Input: part model. Units: mm. Frame: model coordinates. A direction names the side the tool comes from. Round coordinates to 2 decimals unless told otherwise and drop trailing zeros. Order: outer loops, then holes, each group sorted by start corner. A loop starts at its lowest first (then second) coordinate and runs counter-clockwise, first axis right, second up. Notation, with made-up numbers: (-16.75, 58.25) - (-6.75, 58.25) arc R21 ccw to (-6.75, 64.25) - close; hole circle Ø6 at (57.25, -35.5). An arc over 180 degrees is marked (long way). One line per item, written item: value. Start each with the question number.
from build123d import *

# Parameters (mm, degrees)
SKETCH2_R           = 5.55625
BOSS_EXTRUDE1_DEPTH = 15
CHAMFER1_SIZE       = 0.5


with BuildPart() as part:
    # Sketch1 → Revolve1 (revolve)
    with BuildSketch(Plane(origin=(0, 0, 0), x_dir=(1, 0, 0), z_dir=(0, 1, 0))):
        Polygon((1, 25), (2, 25), (2, 15), (7.9375, 15), (7.9375, 0), (5.55625, 0), (5.55625, 12), (1, 12), align=None)
    revolve(axis=Axis((0, 0, 0), (0, 0, -1)))

    # Sketch2 → Boss-Extrude1 (add, through all)
    with BuildSketch(Plane(origin=(0, 0, -15), x_dir=(-1, 0, 0), z_dir=(0, 0, -1))):
        Polygon((9.165435523, 0), (4.582717762, 7.9375), (-4.582717762, 7.9375), (-9.165435523, 0), (-4.582717762, -7.9375), (4.582717762, -7.9375), align=None)
        with Locations(Location((0, 0, 0), (0, 0, 180))):
            Circle(SKETCH2_R, mode=Mode.SUBTRACT)
    extrude(amount=-BOSS_EXTRUDE1_DEPTH)

    # Chamfer1
    chamfer1_edges = [part.edges().sort_by_distance(p)[0] for p in [
        (-6.874076643, -3.96875, -15),
        (0, -7.9375, -15),
        (6.874076643, -3.96875, -15),
        (6.874076643, 3.96875, -15),
        (0, 7.9375, -15),
        (-6.874076643, 3.96875, -15),
        (-6.874076643, -3.96875, 0),
        (0, -7.9375, 0),
        (6.874076643, -3.96875, 0),
        (6.874076643, 3.96875, 0),
        (0, 7.9375, 0),
        (-6.874076643, 3.96875, 0),
        (-5.55625, 0, 0),
        (-2, 0, -25),
    ]]
    chamfer(chamfer1_edges, length=CHAMFER1_SIZE)


solid = part.part
1. Pull-direction query (Y, two-part tool) for faces 1 (the face through (-6.842, -4.024, -7.598)), 2 (the face through (6.69, 3.79, -0.25)), 3 (the face through (0, 1, -19)), 4 (the face through (0, 2, -20)); classes: released by +Y, released by -Y, zero draft, split by the parting line, or undercut.
2. Section C-C (z = -3.25). Return the cut outline in (x, y), then the cut area to 3 significant figures.
3. Pin query (flat end, axial travel): pin 1 (6 mm diameter, centred on y = 4, z = -15.5, fed in from -X); pin 2 (1 mm diameter, centred on x = -6.5, y = 5.5, fed in from +Z); pin 3 (1.5 mm diameter, centred on x = 3.5, y = 0.5, fed in from -Z); pin 4 (3 mm diameter, centred on x = 0, y = 0, fed in from -Z). Return the tip coordinate at first contact, or that it passes through.
4. Section D-D (y = 6.5). Return the cut outline in (x, z).
5. Line query: line 1 (X direction, y = 0, z = -17.75); line 2 (Y direction, x = 0, z = -9.5); line 3 (Z direction, x = -3.25, y = 0.5). Output: solid intervals per line, ascending. Write a range as from..to.
6. Section A-A (z = -12.75). Return the cut outline in (x, y).
7. Set-up query: faces 5 (the face through (-2, 2, -15)), 6 (the face through (5.3, -1.67, -6.33)), 7 (the face through (-6.622, 3.898, -14.754)). Return all of +Z, -Z, +X, -X, +Y, -Y with unobstructed straight access to the full face (end or side cutting, diameter ignored); none if empty.
8. Section B-B (x = 0). Return the cut outline in (y, z), then the cut area to 3 significant figures.
Solved:
1. face 1: released by -Y
1. face 2: released by +Y
1. face 3: undercut
1. face 4: split by the parting line
2. outline: (-9.17, 0) - (-4.58, -7.94) - (4.58, -7.94) - (9.17, 0) - (4.58, 7.94) - (-4.58, 7.94) - close; hole circle Ø11.11 at (0, 0)
2. area: 121 mm²
3. pin 1: stops at x = -8.49
3. pin 2: stops at z = -0.44
3. pin 3: stops at z = -15
3. pin 4: stops at z = -25
4. outline: (-5.41, -14.5) - (-4.84, -15) - (4.84, -15) - (5.41, -14.5) - (5.41, -0.5) - (4.84, 0) - (-4.84, 0) - (-5.41, -0.5) - close
5. line 1: x = -2..-1, 1..2
5. line 2: y = -7.94..-5.56, 5.56..7.94
5. line 3: z = -15..-12
6. outline: (-9.17, 0) - (-4.58, -7.94) - (4.58, -7.94) - (9.17, 0) - (4.58, 7.94) - (-4.58, 7.94) - close; hole circle Ø2 at (0, 0)
7. face 5: -Z
7. face 6: +Z
7. face 7: -Z, -X, +Y
8. outline: (-7.94, -14.5) - (-7.44, -15) - (-2, -15) - (-2, -24.5) - (-1.5, -25) - (-1, -25) - (-1, -12) - (-5.56, -12) - (-5.56, -0.5) - (-6.06, 0) - (-7.44, 0) - (-7.94, -0.5) - close; (1, -25) - (1.5, -25) - (2, -24.5) - (2, -15) - (7.44, -15) - (7.94, -14.5) - (7.94, -0.5) - (7.44, 0) - (6.06, 0) - (5.56, -0.5) - (5.56, -12) - (1, -12) - close
8. area: 118 mm²
